The model under review builds one solid part; all positions refer to its coordinate system, in mm. Face numbers are marked on the shaded views. A direction names the side the tool comes from. Coordinates: 2 decimals unless noted, no trailing zeros. Order: outer loops, then holes, each group sorted by start corner. A loop starts at its lowest first (then second) coordinate and runs counter-clockwise, first axis right, second up. Notation, with made-up numbers: (20, 70) -> (58, 70) arc R21 cw to (58, 86) -> close; hole circle Ø2 at (-21.5, 82.25). An arc over 180 degrees is marked (long way). Use one line per item in the form item = value. Start each with the question number.
(1) Wall thickness on line 1 along Y through (x, z) = (5.45, -4); line 2 along X through (y, z) = (2, -7.5); line 3 along Y through (x, z) = (-2, -7.25): over which ranges is each line inside the solid? List them lowest first.
(2) Take a section at D-D (y = 2.25). State the section outline as (x, z) points.
(3) For the marked faces 1 and 2, list the 3-axis set-ups (+Z, -Z, +X, -X, +Y, -Y) from which the entire face can be reached by the end or side of a thin tool; tool diameter is ignored.
(4) Mouldability with a two-part tool opening along Y and no side actions: class the marked faces 3, 4, 5 and 6 as +Y half, -Y half, draft (parallel to the pull), parting line (faces both ways), or undercut.
(5) Take a section at C-C (x = 0). State the section outline as (y, z) points, then the cut area to 3 significant figures.
(6) Take a section at A-A (z = -4). State the section outline as (x, y) points.
(7) Take a section at B-B (y = 7). State the section outline as (x, z) points, then the cut area to 3 significant figures.
(8) Insertion check: pin 1 Ø1.8 at (x, z) = (0, -7.5) entering from +Y; pin 2 Ø1 at (x, z) = (1.5, 4) entering from +Y; pin 3 Ø2 at (y, z) = (7, 3) entering from -X. Each pin has a flat end and moves straight along its axis. Give the tip position at first contact, or say it passes through.
```python
from build123d import *

# Parameters (mm, degrees)
SKETCH_1_W          = 7
SKETCH_1_H          = 22
SKETCH_1_R          = 1
SKETCH_1_W_2        = 3.5
EXTRUDE_1_DEPTH     = 3
SKETCH_2_W          = 3
SKETCH_2_H          = 22
EXTRUDE_2_DEPTH     = 8
SKETCH_3_R          = 1.5
CUT_EXTRUDE_1_DEPTH = 8
FILLET_1_R          = 2
FILLET_2_R          = 1


with BuildPart() as part:
    # 草图1 → 凸台-拉伸1 (new body)
    # profile 1 of 2: a face of its own
    with BuildSketch(Plane(origin=(0, 0, 0), x_dir=(1, 0, 0), z_dir=(0, 1, 0))):
        Rectangle(SKETCH_1_W, SKETCH_1_H)
        with Locations(Location((0, 7.5, 0), (0, 0, 270))):
            Circle(SKETCH_1_R, mode=Mode.SUBTRACT)
        with Locations(Location((0, -7.5, 0), (0, 0, 270))):
            Circle(SKETCH_1_R, mode=Mode.SUBTRACT)
    # profile 2 of 2: a face of its own
    with BuildSketch(Plane(origin=(0, 0, 0), x_dir=(1, 0, 0), z_dir=(0, 1, 0))):
        with Locations((5.25, 0)):
            Rectangle(SKETCH_1_W_2, SKETCH_1_H)
    extrude(amount=EXTRUDE_1_DEPTH)

    # 草图2 → 凸台-拉伸2 (add)
    with BuildSketch(Plane(origin=(0, 3, 0), x_dir=(1, 0, 0), z_dir=(0, 1, 0))):
        with Locations((5.5, 0)):
            Rectangle(SKETCH_2_W, SKETCH_2_H)
    extrude(amount=EXTRUDE_2_DEPTH)

    # 草图3 → 切除-拉伸1 (cut)
    with BuildSketch(Plane.ZY.offset(-4)):
        with Locations((4, 7)):
            Circle(SKETCH_3_R)
        with Locations(Location((-4, 7, 0), (0, 0, 180))):
            Circle(SKETCH_3_R)
    extrude(amount=-CUT_EXTRUDE_1_DEPTH, mode=Mode.SUBTRACT)

    # 圆角1
    fillet_1_edges = [part.edges().sort_by_distance(p)[0] for p in [
        (-3.5, 1.5, 11),
        (-3.5, 1.5, -11),
        (5.5, 11, -11),
        (5.5, 11, 11),
    ]]
    fillet(fillet_1_edges, radius=FILLET_1_R)

    # 圆角2
    fillet_2_edges = [part.edges().sort_by_distance(p)[0] for p in [
        (7, 0, 0),
        (4, 3, 0),
    ]]
    fillet(fillet_2_edges, radius=FILLET_2_R)


solid = part.part
```
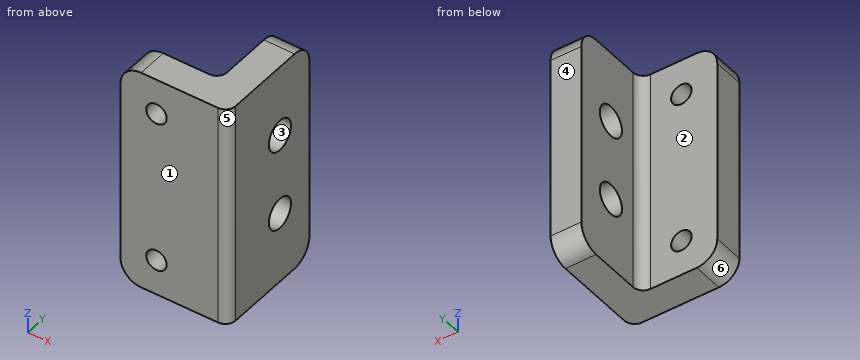
Findings:
q1.line_1 = 0 to 5.5, 8.5 to 11
q1.line_2 = -3.5 to -1, 1 to 7
q1.line_3 = 0 to 3
q2.outline = (-3.5, -9) arc R2 ccw to (-1.5, -11) -> (7, -11) -> (7, 11) -> (-1.5, 11) arc R2 ccw to (-3.5, 9) -> close; hole circle Ø2 at (0, -7.5); hole circle Ø2 at (0, 7.5)
q3.face_1 = +Z, -Z, +X, -X, -Y
q3.face_2 = +Z, -Z, -X, +Y
q4.face_3 = undercut
q4.face_4 = +Y half
q4.face_5 = -Y half
q4.face_6 = draft
q5.outline = (0, -11) -> (3, -11) -> (3, -8.5) -> (0, -8.5) -> close; (0, -6.5) -> (3, -6.5) -> (3, 6.5) -> (0, 6.5) -> close; (0, 8.5) -> (3, 8.5) -> (3, 11) -> (0, 11) -> close
q5.area = 54.0 mm²
q6.outline = (-3.5, 0) -> (6, 0) arc R1 ccw to (7, 1) -> (7, 5.5) -> (4, 5.5) -> (4, 4) arc R1 cw to (3, 3) -> (-3.5, 3) -> close; (4, 8.5) -> (7, 8.5) -> (7, 11) -> (4, 11) -> close
q7.outline = (4, -11) -> (7, -11) -> (7, -5.5) -> (4, -5.5) -> close; (4, -2.5) -> (7, -2.5) -> (7, 2.5) -> (4, 2.5) -> close; (4, 5.5) -> (7, 5.5) -> (7, 11) -> (4, 11) -> close
q7.area = 48.0 mm²
q8.pin_1 = through
q8.pin_2 = 3
q8.pin_3 = 4
